Part model, mm, in its own coordinate system. A direction names the side the tool comes from. Round coordinates to 2 decimals unless told otherwise and drop trailing zeros. Write each loop counter-clockwise with the first axis right and the second up, starting at its lowest first coordinate (ties: lowest second). Pieces come first, ordered by that corner, then holes. Notation, with made-up numbers: M -11.75,26.25 L 22.25,26.25 A26 cw 22.25,55.25 Z; hole C 36.25,-11 d5. An arc over 180 degrees is marked long. One line per question, with ' | ' between items. Start each with the question number.
1) Mould opens along Y. For faces 4 (the face through (-43, -25, 45)), 5 (the face through (-43.75, -18.85, 45.07)), 6 (the face through (47.5, -12, 45)) say: pulls with the +Y half, pulls with the -Y half, needs draft (parallel to the pull), parting line crosses it, or undercut.
2) Tool access for faces 1 (the face through (97, 27, 25)), 2 (the face through (-43, -12, 40)), 3 (the face through (-37.5, -12, 45)): list every direction of +Z, -Z, +X, -X, +Y, -Y with a clear straight run to the whole face (end or side of a thin tool).
3) Saw through at C-C (x = -30). List the corners of the cut face in (y, z), plus the area to 3 significant figures.
4) Drop flat-ended pins along their axis: pin 1 Ø6 at (x, z) = (-37.5, 15) entering from -Y; pin 2 Ø12 at (y, z) = (-5.5, 10) entering from +X; pin 3 Ø2 at (x, z) = (70, 15) entering from -Y; pin 4 Ø5.5 at (x, z) = (-70, 35) entering from +Y. Give the stop position or say it passes through.
5) Saw through at B-B (y = 34.5). List the corners of the cut face in (x, z), plus the area to 3 significant figures.
6) Saw through at A-A (y = -10). List the corners of the cut face in (x, z).
7) Wall check: probe 1 along Z at (x, y) = (-70, 2.15); probe 2 along Y at (x, z) = (-42.5, 49); probe 3 along X at (y, z) = (0.6, 35). Give the ranges that are in metal, low to high. Write a range as [from, to].
```python
from build123d import *

# Parameters (mm, degrees)
BOX_FOOTPRINT_200_X_50_MM_W                     = 200
BOX_FOOTPRINT_200_X_50_MM_H                     = 50
BOX_HEIGHT_50_MM_DEPTH                          = 50
REAR_OPENING_194_X_44_MM_W                      = 194
REAR_OPENING_194_X_44_MM_H                      = 44
REAR_CAVITY_WALL_3_MM_DEPTH                     = 47
TWO_SQUARE_ARMS_10_X_10_PITCH_85_MM_W           = 10
TWO_SQUARE_ARMS_10_X_10_PITCH_85_MM_H           = 10
FORWARD_SQUARE_ARMS_25_MM_DEPTH                 = 25
TEMPORARY_CHASSIS_HOLES_140_X_20_MM_R           = 1.7
F_4X_M3_CLEARANCE_DIAMETER_3_4_MM_DEPTH         = 3
PCB_REAR_PAIR_PITCH_85_MM_R                     = 1.7
F_2X_ROOF_HOLES_DIAMETER_3_4_MM_DEPTH           = 3
PCB_FRONT_PAIR_ROW_SPACING_60_MM_R              = 1.7
F_2X_ARM_HOLES_THROUGH_TOP_AND_BOTTOM_3_4_DEPTH = 10


with BuildPart() as part:
    # Box footprint 200 x 50 mm → Box height 50 mm (new body)
    with BuildSketch(Plane.XY):
        with Locations((0, 25)):
            Rectangle(BOX_FOOTPRINT_200_X_50_MM_W, BOX_FOOTPRINT_200_X_50_MM_H)
    extrude(amount=BOX_HEIGHT_50_MM_DEPTH)

    # Rear opening 194 x 44 mm → Rear cavity - wall 3 mm (cut)
    with BuildSketch(Plane(origin=(0, 50, 0), x_dir=(1, 0, 0), z_dir=(0, 1, 0))):
        with Locations((0, -25)):
            Rectangle(REAR_OPENING_194_X_44_MM_W, REAR_OPENING_194_X_44_MM_H)
    extrude(amount=-REAR_CAVITY_WALL_3_MM_DEPTH, mode=Mode.SUBTRACT)

    # Two square arms 10 x 10 - pitch 85 mm → Forward square arms 25 mm (add)
    with BuildSketch(Plane.XZ):
        with Locations((-42.5, 45)):
            Rectangle(TWO_SQUARE_ARMS_10_X_10_PITCH_85_MM_W, TWO_SQUARE_ARMS_10_X_10_PITCH_85_MM_H)
        with Locations((42.5, 45)):
            Rectangle(TWO_SQUARE_ARMS_10_X_10_PITCH_85_MM_W, TWO_SQUARE_ARMS_10_X_10_PITCH_85_MM_H)
    extrude(amount=FORWARD_SQUARE_ARMS_25_MM_DEPTH)

    # Temporary chassis holes - 140 x 20 mm → 4x M3 clearance diameter 3.4 mm (cut)
    with BuildSketch(Plane.XZ):
        with Locations(Location((-70, 15, 0), (0, 0, 270))):
            Circle(TEMPORARY_CHASSIS_HOLES_140_X_20_MM_R)
        with Locations(Location((-70, 35, 0), (0, 0, 270))):
            Circle(TEMPORARY_CHASSIS_HOLES_140_X_20_MM_R)
        with Locations(Location((70, 15, 0), (0, 0, 270))):
            Circle(TEMPORARY_CHASSIS_HOLES_140_X_20_MM_R)
        with Locations(Location((70, 35, 0), (0, 0, 270))):
            Circle(TEMPORARY_CHASSIS_HOLES_140_X_20_MM_R)
    extrude(amount=-F_4X_M3_CLEARANCE_DIAMETER_3_4_MM_DEPTH, mode=Mode.SUBTRACT)

    # PCB rear pair - pitch 85 mm → 2x roof holes diameter 3.4 mm (cut)
    with BuildSketch(Plane.XY.offset(50)):
        with Locations((-42.5, 40)):
            Circle(PCB_REAR_PAIR_PITCH_85_MM_R)
        with Locations((42.5, 40)):
            Circle(PCB_REAR_PAIR_PITCH_85_MM_R)
    extrude(amount=-F_2X_ROOF_HOLES_DIAMETER_3_4_MM_DEPTH, mode=Mode.SUBTRACT)

    # PCB front pair - row spacing 60 mm → 2x arm holes through top and bottom 3.4 mm (cut)
    with BuildSketch(Plane.XY.offset(50)):
        with Locations((-42.5, -20)):
            Circle(PCB_FRONT_PAIR_ROW_SPACING_60_MM_R)
        with Locations((42.5, -20)):
            Circle(PCB_FRONT_PAIR_ROW_SPACING_60_MM_R)
    extrude(amount=-F_2X_ARM_HOLES_THROUGH_TOP_AND_BOTTOM_3_4_DEPTH, mode=Mode.SUBTRACT)


solid = part.part
```
Answer key:
1) face 4: pulls with the -Y half | face 5: undercut | face 6: needs draft
2) face 1: +Y | face 2: -Z, +X, -X, -Y | face 3: +Z, -Z, -Y
3) outline: M 0,0 L 50,0 L 50,3 L 3,3 L 3,47 L 50,47 L 50,50 L 0,50 Z | area: 432 mm2
4) pin 1: stops at y = 0 | pin 2: stops at x = 100 | pin 3: passes through | pin 4: stops at y = 3
5) outline: M -100,0 L 100,0 L 100,50 L -100,50 Z; hole M -97,3 L 97,3 L 97,47 L -97,47 Z | area: 1,460 mm2
6) outline: M -47.5,40 L -37.5,40 L -37.5,50 L -47.5,50 Z; M 37.5,40 L 47.5,40 L 47.5,50 L 37.5,50 Z
7) probe 1: z = [0, 13.3], [16.7, 33.3], [36.7, 50] | probe 2: y = [-25, -21.7], [-18.3, 38.3], [41.7, 50] | probe 3: x = [-100, -71.7], [-68.3, 68.3], [71.7, 100]
